Source: CAD feature listing. Evaluate the final solid. Frame: model axes, mm. A direction names the side the tool comes from. Give positions to 0.01 mm unless a question says otherwise; leave off trailing zeros. Order: outer loops, then holes, each group sorted by start corner. A loop starts at its lowest first (then second) coordinate and runs counter-clockwise, first axis right, second up.
from build123d import *

# Parameters (mm, degrees)
F2_R    = 2
F3_SIZE = 3


with BuildPart() as f1:
    # F0 (on Front) → F1 (revolve)
    with BuildSketch(Plane.XZ):
        with BuildLine():
            Line((36.9, 20), (36.9, 2))
            Line((36.9, 2), (0, 2))
            Line((0, 2), (0, 1))
            add(Edge.make_bspline(
                [(29.7, 0), (15.418199, 0), (18.330893, 1), (0, 1)],
                knots=[0, 0, 0, 0, 29.71683, 29.71683, 29.71683, 29.71683], degree=3))
            Line((29.7, 0), (37.7, 0))
            Line((37.7, 0), (37.7, 20))
            Line((37.7, 20), (36.9, 20))
        make_face()
    revolve(axis=Axis((0, 0, 19.229219), (0, 0, 1)))

    # F2
    f2_edges = [f1.edges().sort_by_distance(p)[0] for p in [
        (-36.9, 0, 2),
    ]]
    fillet(f2_edges, radius=F2_R)

    # F3
    f3_edges = [f1.edges().sort_by_distance(p)[0] for p in [
        (-37.7, 0, 0),
    ]]
    chamfer(f3_edges, length=F3_SIZE)


solid = f1.part
1) Reachability of faces 4 (the face through (0, 0, 2)), 5 (the face through (28, -25, 20)) from +Z, -Z, +X, -X, +Y, -Y: full face, straight path, thin tool, end or side. Return the list, or none.
Checks:
face 4: +Z
face 5: +Z, +X, -X, +Y, -Y
2) Pull-direction query (Y, two-part tool) for faces 1 (the face through (-27.652, -21.203, 0.146)), 2 (the face through (19.837, 31.114, 11.888)), 3 (the face through (-26, 16, 0)); classes: +Y half, -Y half, draft (parallel to the pull), parting line (faces both ways), or undercut.
Checks:
face 1: parting line
face 2: undercut
face 3: draft
3) Ray query, L1, parallel to Y at x = 0, z = 15.5; L2, parallel to Z at x = -33, y = 6.5; L3, parallel to Y at x = -10.5, z = 11.5. Return the intervals inside material, ascending.
Checks:
L1: y = -37.7 to -36.9, 36.9 to 37.7
L2: z = 0 to 2
L3: y = -36.21 to -35.37, 35.37 to 36.21
4) Section query A-A on z = 15. Output: boundary loops of the cut face in (x, y).
Checks:
outline: circle Ø75.4 at (0, 0); hole circle Ø73.8 at (0, 0)
5) First-contact query: pin 1 Ø12 at (x, y) = (-3, 10) entering from +Z; pin 2 Ø1.5 at (x, z) = (-26, 16.5) entering from -Y; pin 3 Ø1.5 at (x, y) = (7, -4) entering from -Z; pin 4 Ø2 at (x, y) = (-28.5, -21) entering from -Z. Flat tips, straight axial feed; report the tip coordinate or a pass-through.
Checks:
pin 1: stops at z = 2
pin 2: stops at y = -28
pin 3: stops at z = 0.89
pin 4: stops at z = 0
